Design review of the part built by this model. Coordinates are the model's own, in mm. Face numbers are marked on the shaded views. A direction names the side the tool comes from. Coordinates: 2 decimals unless noted, no trailing zeros. Write each loop counter-clockwise with the first axis right and the second up, starting at its lowest first coordinate (ties: lowest second). Pieces come first, ordered by that corner, then holes.
Q1. Mouldability with a two-part tool opening along X and no side actions: class the marked faces 1, 2 and 3 as pulls with the +X half, pulls with the -X half, needs draft (parallel to the pull), parting line crosses it, or undercut.
Q2. Insertion check: pin 1 (4 mm diameter, centred on x = 5.94, z = -5.94, fed in from -Y); pin 2 (7 mm diameter, centred on x = -5.94, z = 5.94, fed in from -Y); pin 3 (7 mm diameter, centred on x = -8.39, z = 0, fed in from +Y); pin 4 (6 mm diameter, centred on y = 1.5, z = -4.5, fed in from -X). Each pin has a flat end and moves straight along its axis. Give the tip position at first contact, or say it passes through.
Q3. Machinability: for the marked faces 4 and 5, which of the approach directions +Z, -Z, +X, -X, +Y, -Y give a long, thin tool a straight path to every point of the face, cutting with its end or side? Answer none if there is none.
Q4. Take a section at B-B (y = 3.25). Give the boundary of the cut face in (x, z).
Q5. Take a section at A-A (z = 0). State how many separate pieces and enclosed holes the cut face has, and give its area (3 significant figures).
Q6. For probe 1 along Z at (x, y) = (0, -1.2); probe 2 along Z at (x, y) = (-4, -0.25); probe 3 along Y at (x, z) = (-13, -4.5), list the stretches that pass through material, from the lowest coordinate up.
```python
from build123d import *

# Parameters (mm, degrees)
F0_R      = 17
F1_DEPTH  = 2.5
F2_R      = 2
F4_R      = 15
F4_R_2    = 11.25
F6_DEPTH  = 1
F5_R      = 5
F8_DEPTH  = 1
F7_R      = 2.1850910156
F9_DEPTH  = 25.4
F10_R     = 2.6038843179
F11_DEPTH = 1
F12_R     = 0.6358860885
F13_DEPTH = 0.5
F14_DEPTH = 0.5
F15_R     = 2.3875943528
F16_DEPTH = 7.5


# Not quite as in the source:
# - a fillet or chamfer that OpenCascade refuses, or shapes differently, is made with other operations: its cross-section is extruded or revolved along the edge and cut away or added


with BuildPart() as f1:
    # F0 (on Front) → F1 (new body)
    with BuildSketch(Plane.XZ):
        Circle(F0_R)
    extrude(amount=F1_DEPTH)

    # F2
    f2_edges = [f1.edges().sort_by_distance(p)[0] for p in [
        (-17, -2.5, 0),
    ]]
    fillet(f2_edges, radius=F2_R)

    # F3: fillet of radius 2 on 1 edges, made by hand

    # F3_s1 → F3_t2 (revolve, cut)
    with BuildSketch(Plane.XY):
        with BuildLine():
            ThreePointArc((17, -0.5), (16.3842311257, -0.1291713066), (15.6771243445, 0))
            Line((15.6771243445, 0), (17, 0))
            Line((17, 0), (17, -0.5))
        make_face()
    revolve(axis=Axis((0, 0, 0), (0, -1, 0)), mode=Mode.SUBTRACT)

    # F4 (on face) → F6 (cut)
    with BuildSketch(Plane.XZ.offset(2.5)):
        Circle(F4_R)
        Circle(F4_R_2, mode=Mode.SUBTRACT)
    extrude(amount=-F6_DEPTH, mode=Mode.SUBTRACT)

    # F5 (on face) → F8 (join)
    with BuildSketch(Plane.XZ.offset(2.5)):
        Circle(F5_R)
    extrude(amount=F8_DEPTH)

    # F7 (on face) → F9 (cut)
    with BuildSketch(Plane.XZ.offset(2.5)):
        with Locations((0, 8.3935074508)):
            Circle(F7_R)
        with Locations((5.9351060364, 5.9351060364)):
            Circle(F7_R)
        with Locations((8.3935074508, 0)):
            Circle(F7_R)
        with Locations((5.9351060364, -5.9351060364)):
            Circle(F7_R)
        with Locations((0, -8.3935074508)):
            Circle(F7_R)
        with Locations((-5.9351060364, -5.9351060364)):
            Circle(F7_R)
        with Locations((-8.3935074508, 0)):
            Circle(F7_R)
        with Locations((-5.9351060364, 5.9351060364)):
            Circle(F7_R)
    extrude(amount=-F9_DEPTH, mode=Mode.SUBTRACT)

    # F10 (on face) → F11 (join)
    with BuildSketch(Plane.XZ.offset(3.5)):
        Circle(F10_R)
    extrude(amount=F11_DEPTH)

    # F12 (on face) → F13 (join)
    with BuildSketch(Plane.XZ.offset(3.5)):
        with Locations((-2.3013945397, 3.1675978363)):
            Circle(F12_R)
        with Locations((0, 3.915366251)):
            Circle(F12_R)
        with Locations((2.3013945397, 3.1675978363)):
            Circle(F12_R)
        with Locations((3.7237345867, 1.2099147108)):
            Circle(F12_R)
        with Locations((3.7237345867, -1.2099147108)):
            Circle(F12_R)
        with Locations((2.3013945397, -3.1675978363)):
            Circle(F12_R)
        with Locations((0, -3.915366251)):
            Circle(F12_R)
        with Locations((-2.3013945397, -3.1675978363)):
            Circle(F12_R)
        with Locations((-3.7237345867, -1.2099147108)):
            Circle(F12_R)
        with Locations((-3.7237345867, 1.2099147108)):
            Circle(F12_R)
    extrude(amount=F13_DEPTH)

    # F14 (add): faces of the model
    f14_faces = [f1.faces().sort_by_distance(p)[0] for p in [
        (3.7237345867, -4, 1.2099147108),
        (2.3013945397, -4, 3.1675978363),
        (0, -4, 3.915366251),
        (-2.3013945397, -4, 3.1675978363),
        (-3.7237345867, -4, 1.2099147108),
        (-3.7237345867, -4, -1.2099147108),
        (-2.3013945397, -4, -3.1675978363),
        (0, -4, -3.915366251),
        (2.3013945397, -4, -3.1675978363),
        (3.7237345867, -4, -1.2099147108),
    ]]
    extrude(f14_faces, amount=F14_DEPTH)

    # F15 (on face) → F16 (join)
    with BuildSketch(Plane(origin=(0, 0, 0), x_dir=(-1, 0, 0), z_dir=(0, 1, 0))):
        Circle(F15_R)
    extrude(amount=F16_DEPTH)


solid = f1.part
```
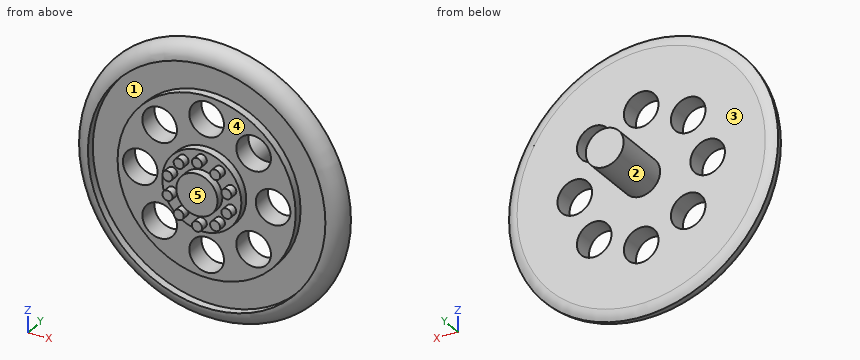
Response:
1. face 1: undercut
1. face 2: parting line crosses it
1. face 3: needs draft
2. pin 1: passes through
2. pin 2: stops at y = -3.5
2. pin 3: stops at y = 0
2. pin 4: stops at x = -16.85
3. face 4: -Y
3. face 5: +Z, -Z, +X, -X, -Y
4. outline: circle Ø4.78 at (0, 0)
5. separate pieces: 3
5. enclosed holes: 0
5. area: 105 mm2
6. probe 1: z = -16.87 to -10.58, -6.21 to 6.21, 10.58 to 16.87
6. probe 2: z = -16.16 to -6.95, -4.92 to 4.92, 6.95 to 16.16
6. probe 3: y = -1.5 to 0
